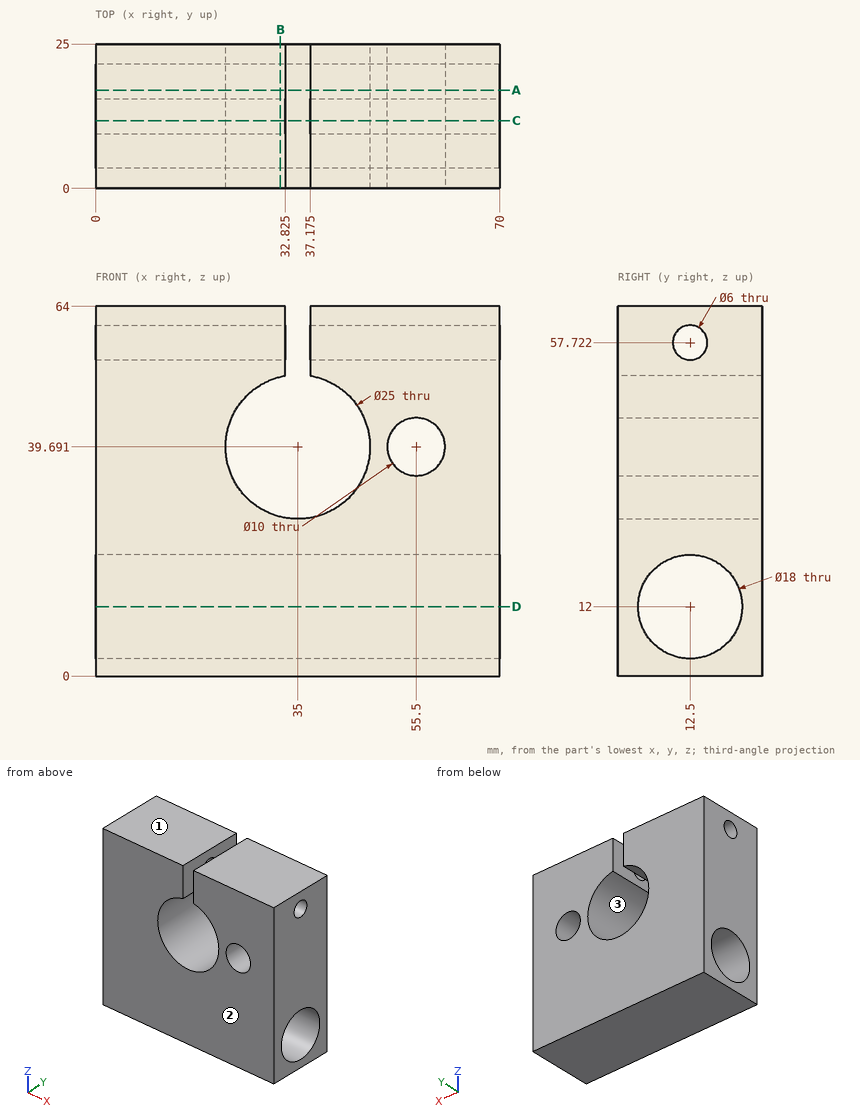
Print and shaded views of the part. All mm, measured from the part's lowest x, y and z. Coordinates: 2 decimals unless noted, no trailing zeros. Order: outer loops, then holes, each group sorted by start corner. A loop starts at its lowest first (then second) coordinate and runs counter-clockwise, first axis right, second up. Notation, with made-up numbers: M 61,71.5 L 74,71.5 A21 ccw 74,104.5 Z; hole C -18.5,-1.5 d8. An arc over 180 degrees is marked long. Answer as CSV lines item,"result".
1) Drill centre lines: L1, parallel to Z at x = 58.5, y = 12.5; L2, parallel to X at y = 1.5, z = 53 (1 decimal); L3, parallel to Z at x = 55.5, y = 6.75 (1 decimal). Where is each one in solid material? Low to high. Write a range as from..to.
Verdict:
L1,"0..3, 21..35.69, 43.69..54.72, 60.72..64"
L2,"0..32.8, 37.2..70"
L3,"0..5.1, 18.9..34.7, 44.7..64"
2) Cut at D-D (z = 12). List the corners of the cut face in (x, y), then the cut area to 3 significant figures.
Verdict:
outline,"M 0,0 L 70,0 L 70,3.5 L 0,3.5 Z; M 0,21.5 L 70,21.5 L 70,25 L 0,25 Z"
area,"490 mm2"
3) Cut at C-C (y = 11.75). List the corners of the cut face in (x, z) (1 decimal), then the cut area to 3 significant figures.
Verdict:
outline,"M 0,0 L 70,0 L 70,3 L 0,3 Z; M 0,21 L 70,21 L 70,54.8 L 37.2,54.8 L 37.2,52 A12.5 cw long 32.8,52 L 32.8,54.8 L 0,54.8 Z; M 0,60.6 L 32.8,60.6 L 32.8,64 L 0,64 Z; M 37.2,60.6 L 70,60.6 L 70,64 L 37.2,64 Z; hole C 55.5,39.7 d10"
area,"2,220 mm2"
4) Flat gauge pins, fed straight in: P1, Ø5, axis at x = 42.5, y = 15, coming from the -Z side; P2, Ø6, axis at x = 55.5, z = 39.69, coming from the -Y side. Where does each tip first touch, or does it go through?
Verdict:
P1,"z = 0"
P2,"through"
5) Mould opens along Z. For the marked faces 1, 2 and 3 say: released by +Z, released by -Z, zero draft, split by the parting line, or undercut.
Verdict:
face 1,"released by +Z"
face 2,"zero draft"
face 3,"undercut"
6) Cut at B-B (x = 32). List the corners of the cut face in (y, z) (1 decimal).
Verdict:
outline,"M 0,0 L 25,0 L 25,27.6 L 0,27.6 Z; M 0,51.8 L 25,51.8 L 25,64 L 0,64 Z; hole C 12.5,12 d18; hole C 12.5,57.7 d6"
7) Cut at A-A (y = 17). List the corners of the cut face in (x, z) (1 decimal), then the cut area to 3 significant figures.
Verdict:
outline,"M 0,0 L 70,0 L 70,4.2 L 0,4.2 Z; M 0,19.8 L 70,19.8 L 70,64 L 37.2,64 L 37.2,52 A12.5 cw long 32.8,52 L 32.8,64 L 0,64 Z; hole C 55.5,39.7 d10"
area,"2,770 mm2"
